Source: CAD feature listing. Evaluate the final solid. Frame: model axes, mm. Face numbers are marked on the shaded views. Coordinates: 2 decimals unless noted, no trailing zeros. Write each loop counter-clockwise with the first axis right and the second up, starting at its lowest first coordinate (ties: lowest second). Pieces come first, ordered by that corner, then holes. Notation, with made-up numbers: (-39.5, -5.75) -> (-30.5, -5.75) arc R16 ccw to (-30.5, 5.25) -> close; hole circle Ø8 at (52.25, 26). An arc over 180 degrees is marked (long way). One line per item, written item: value. Start each with the question number.
1. Section query B-B, the plane z = -12.5. Output: boundary loops of the cut face in (x, y) (3 decimals), and give its area (3 significant figures).
2. Section query A-A, the plane x = 55.4. Output: boundary loops of the cut face in (y, z) (3 decimals), and give its area (3 significant figures).
3. Section query C-C, the plane z = -23. Output: boundary loops of the cut face in (x, y) (3 decimals).
4. Mould query, pull axis Z, two halves, no side actions, for the marked faces 1 and 2. Classes: released by +Z, released by -Z, zero draft, split by the parting line, or undercut.
5. Line query: line 1 (X direction, y = -0.05, z = -74.5); line 2 (X direction, y = -3.5, z = -37); line 3 (Z direction, x = 18, y = -2.5). Output: solid intervals per line, ascending.
6. First-contact query: P1, Ø3.5, axis at x = 30, z = -54.5, coming from the +Y side (3 decimals); P2, Ø10, axis at x = 69, z = -76, coming from the -Y side (3 decimals); P3, Ø3.5, axis at x = 36.9, z = -2.5, coming from the +Y side; P4, Ø2, axis at x = 36.5, z = 3.5, coming from the -Y side (3 decimals). Flat tips, straight axial feed; report the tip coordinate or a pass-through.
from build123d import *

# Parameters (mm, degrees)
SKETCH1_W           = 85.8
SKETCH1_H           = 92.5
SKETCH1_R           = 2.05
BOSS_EXTRUDE1_DEPTH = 3.175
SKETCH2_W           = 85.8
SKETCH2_H           = 92.5
SKETCH2_R           = 1.35
SKETCH2_R_2         = 3.35
BOSS_EXTRUDE2_DEPTH = 1.905
BOSS_EXTRUDE3_START = 1
SKETCH2_3_W         = 85.8
SKETCH2_3_H         = 92.5
SKETCH2_3_R         = 1.35
SKETCH2_3_R_2       = 3.35
BOSS_EXTRUDE3_DEPTH = 1
SKETCH3_W           = 85.8
SKETCH3_H           = 92.5
SKETCH3_W_2         = 75.8
SKETCH3_H_2         = 82.5
BOSS_EXTRUDE4_DEPTH = 4.55
SKETCH4_W           = 14
SKETCH4_H           = 6.75
CUT_EXTRUDE1_DEPTH  = 118.864146478
SKETCH5_W           = 10
SKETCH5_H           = 6
CUT_EXTRUDE2_DEPTH  = 118.864146478
BOSS_EXTRUDE5_DEPTH = 5
FILLET1_R           = 2.5
FILLET2_R           = 2.5
FILLET3_R           = 2.5
FILLET4_R           = 2.5
FILLET5_R           = 2.5


with BuildPart() as part:
    # Sketch1 → Boss-Extrude1 (new body)
    with BuildSketch(Plane(origin=(0, 0, 0), x_dir=(1, 0, 0), z_dir=(0, 1, 0))):
        with Locations((36.9, 40.25)):
            Rectangle(SKETCH1_W, SKETCH1_H)
        with Locations(Location((2.5, 12.5, 0), (0, 0, 270))):
            Circle(SKETCH1_R, mode=Mode.SUBTRACT)
        with Locations(Location((18.4, 2.5, 0), (0, 0, 270))):
            Circle(SKETCH1_R, mode=Mode.SUBTRACT)
        with Locations(Location((36.9, 2.5, 0), (0, 0, 270))):
            Circle(SKETCH1_R, mode=Mode.SUBTRACT)
        with Locations(Location((55.4, 2.5, 0), (0, 0, 270))):
            Circle(SKETCH1_R, mode=Mode.SUBTRACT)
        with Locations(Location((29.3, 55.1, 0), (0, 0, 270))):
            Circle(SKETCH1_R, mode=Mode.SUBTRACT)
        with Locations(Location((70.8, 74.5, 0), (0, 0, 270))):
            Circle(SKETCH1_R, mode=Mode.SUBTRACT)
    extrude(amount=BOSS_EXTRUDE1_DEPTH)

    # Sketch2 → Boss-Extrude2 (add)
    # profile 1 of 2: a face of its own
    with BuildSketch(Plane(origin=(0, 0, 0), x_dir=(1, 0, 0), z_dir=(0, 1, 0))):
        with Locations((36.9, 40.25)):
            Rectangle(SKETCH2_W, SKETCH2_H)
        with Locations(Location((2.5, 12.5, 0), (0, 0, 270))):
            Circle(SKETCH2_R, mode=Mode.SUBTRACT)
        with Locations(Location((18.4, 2.5, 0), (0, 0, 270))):
            Circle(SKETCH2_R, mode=Mode.SUBTRACT)
        with Locations(Location((36.9, 2.5, 0), (0, 0, 270))):
            Circle(SKETCH2_R, mode=Mode.SUBTRACT)
        with Locations(Location((55.4, 2.5, 0), (0, 0, 270))):
            Circle(SKETCH2_R, mode=Mode.SUBTRACT)
        with Locations(Location((70.8, 74.5, 0), (0, 0, 270))):
            Circle(SKETCH2_R, mode=Mode.SUBTRACT)
        with BuildLine():
            Line((65.8, 74.5), (65.8, 81.5))
            Line((65.8, 81.5), (-1, 81.5))
            Line((-1, 81.5), (-1, 17.5))
            Line((-1, 17.5), (2.5, 17.5))
            ThreePointArc((2.5, 17.5), (7.5, 12.5), (2.5, 7.5))
            Line((2.5, 7.5), (-1, 7.5))
            Line((-1, 7.5), (-1, -1))
            Line((-1, -1), (13.4, -1))
            Line((13.4, -1), (13.4, 2.5))
            ThreePointArc((13.4, 2.5), (18.4, 7.5), (23.4, 2.5))
            Line((23.4, 2.5), (23.4, -1))
            Line((23.4, -1), (31.9, -1))
            Line((31.9, -1), (31.9, 2.5))
            ThreePointArc((31.9, 2.5), (36.9, 7.5), (41.9, 2.5))
            Line((41.9, 2.5), (41.9, -1))
            Line((41.9, -1), (50.4, -1))
            Line((50.4, -1), (50.4, 2.5))
            ThreePointArc((50.4, 2.5), (55.4, 7.5), (60.4, 2.5))
            Line((60.4, 2.5), (60.4, -1))
            Line((60.4, -1), (74.8, -1))
            Line((74.8, -1), (74.8, 69.5))
            Line((74.8, 69.5), (70.8, 69.5))
            ThreePointArc((70.8, 69.5), (67.264466094, 70.964466094), (65.8, 74.5))
        make_face(mode=Mode.SUBTRACT)
    # profile 2 of 2: a face of its own
    with BuildSketch(Plane(origin=(0, 0, 0), x_dir=(1, 0, 0), z_dir=(0, 1, 0))):
        with Locations(Location((29.3, 55.1, 0), (0, 0, 270))):
            Circle(SKETCH2_R_2)
        with Locations(Location((29.3, 55.1, 0), (0, 0, 270))):
            Circle(SKETCH2_R, mode=Mode.SUBTRACT)
    extrude(amount=-BOSS_EXTRUDE2_DEPTH)

    # Sketch2_3 → Boss-Extrude3 (add)
    # profile 1 of 2: a face of its own
    with BuildSketch(Plane(origin=(0, 0, 0), x_dir=(1, 0, 0), z_dir=(0, 1, 0)).offset(BOSS_EXTRUDE3_START)):
        with Locations((36.9, 40.25)):
            Rectangle(SKETCH2_3_W, SKETCH2_3_H)
        with Locations(Location((2.5, 12.5, 0), (0, 0, 270))):
            Circle(SKETCH2_3_R, mode=Mode.SUBTRACT)
        with Locations(Location((18.4, 2.5, 0), (0, 0, 270))):
            Circle(SKETCH2_3_R, mode=Mode.SUBTRACT)
        with Locations(Location((36.9, 2.5, 0), (0, 0, 270))):
            Circle(SKETCH2_3_R, mode=Mode.SUBTRACT)
        with Locations(Location((55.4, 2.5, 0), (0, 0, 270))):
            Circle(SKETCH2_3_R, mode=Mode.SUBTRACT)
        with Locations(Location((70.8, 74.5, 0), (0, 0, 270))):
            Circle(SKETCH2_3_R, mode=Mode.SUBTRACT)
        with BuildLine():
            Line((65.8, 74.5), (65.8, 81.5))
            Line((65.8, 81.5), (-1, 81.5))
            Line((-1, 81.5), (-1, 17.5))
            Line((-1, 17.5), (2.5, 17.5))
            ThreePointArc((2.5, 17.5), (7.5, 12.5), (2.5, 7.5))
            Line((2.5, 7.5), (-1, 7.5))
            Line((-1, 7.5), (-1, -1))
            Line((-1, -1), (13.4, -1))
            Line((13.4, -1), (13.4, 2.5))
            ThreePointArc((13.4, 2.5), (18.4, 7.5), (23.4, 2.5))
            Line((23.4, 2.5), (23.4, -1))
            Line((23.4, -1), (31.9, -1))
            Line((31.9, -1), (31.9, 2.5))
            ThreePointArc((31.9, 2.5), (36.9, 7.5), (41.9, 2.5))
            Line((41.9, 2.5), (41.9, -1))
            Line((41.9, -1), (50.4, -1))
            Line((50.4, -1), (50.4, 2.5))
            ThreePointArc((50.4, 2.5), (55.4, 7.5), (60.4, 2.5))
            Line((60.4, 2.5), (60.4, -1))
            Line((60.4, -1), (74.8, -1))
            Line((74.8, -1), (74.8, 69.5))
            Line((74.8, 69.5), (70.8, 69.5))
            ThreePointArc((70.8, 69.5), (67.264466094, 70.964466094), (65.8, 74.5))
        make_face(mode=Mode.SUBTRACT)
    # profile 2 of 2: a face of its own
    with BuildSketch(Plane(origin=(0, 0, 0), x_dir=(1, 0, 0), z_dir=(0, 1, 0)).offset(BOSS_EXTRUDE3_START)):
        with Locations(Location((29.3, 55.1, 0), (0, 0, 270))):
            Circle(SKETCH2_3_R_2)
        with Locations(Location((29.3, 55.1, 0), (0, 0, 270))):
            Circle(SKETCH2_3_R, mode=Mode.SUBTRACT)
    extrude(amount=-BOSS_EXTRUDE3_DEPTH)

    # Sketch3 → Boss-Extrude4 (add)
    with BuildSketch(Plane(origin=(0, -1.905, 0), x_dir=(-1, 0, 0), z_dir=(0, -1, 0))):
        with Locations((-36.9, 40.25)):
            Rectangle(SKETCH3_W, SKETCH3_H)
        with Locations((-36.9, 40.25)):
            Rectangle(SKETCH3_W_2, SKETCH3_H_2, mode=Mode.SUBTRACT)
    extrude(amount=BOSS_EXTRUDE4_DEPTH)

    # Sketch4 → Cut-Extrude1 (cut, through all)
    with BuildSketch(Plane.XY):
        with Locations((9.15, -6.47)):
            Rectangle(SKETCH4_W, SKETCH4_H)
        with Locations((27.65, -6.47)):
            Rectangle(SKETCH4_W, SKETCH4_H)
        with Locations((46.15, -6.47)):
            Rectangle(SKETCH4_W, SKETCH4_H)
        with Locations((64.65, -6.47)):
            Rectangle(SKETCH4_W, SKETCH4_H)
    extrude(amount=CUT_EXTRUDE1_DEPTH, mode=Mode.SUBTRACT)

    # Sketch5 → Cut-Extrude2 (cut, through all)
    with BuildSketch(Plane.XY):
        with Locations((58, -7.455)):
            Rectangle(SKETCH5_W, SKETCH5_H)
    extrude(amount=-CUT_EXTRUDE2_DEPTH, mode=Mode.SUBTRACT)

    # Sketch6 → Boss-Extrude5 (add)
    with BuildSketch(Plane.ZY.offset(6)):
        with BuildLine():
            Line((-59.6, 0), (-59.6, -8.95))
            Line((-59.6, -8.95), (-59.131128874, -8.95))
            ThreePointArc((-59.131128874, -8.95), (-55.1, -6.45), (-51.068871126, -8.95))
            Line((-51.068871126, -8.95), (-50.6, -8.95))
            Line((-50.6, -8.95), (-50.6, 0))
            Line((-50.6, 0), (-59.6, 0))
        make_face()
    extrude(amount=-BOSS_EXTRUDE5_DEPTH)

    # Fillet1
    fillet1_edges = [part.edges().sort_by_distance(p)[0] for p in [
        (79.8, -1.64, 6),
    ]]
    fillet(fillet1_edges, radius=FILLET1_R)

    # Fillet2
    fillet2_edges = [part.edges().sort_by_distance(p)[0] for p in [
        (79.8, -1.64, -86.5),
    ]]
    fillet(fillet2_edges, radius=FILLET2_R)

    # Fillet3
    fillet3_edges = [part.edges().sort_by_distance(p)[0] for p in [
        (-6, -1.64, -86.5),
    ]]
    fillet(fillet3_edges, radius=FILLET3_R)

    # Fillet4
    fillet4_edges = [part.edges().sort_by_distance(p)[0] for p in [
        (-6, -1.64, 6),
    ]]
    fillet(fillet4_edges, radius=FILLET4_R)

    # Fillet5
    fillet5_edges = [part.edges().sort_by_distance(p)[0] for p in [
        (79.8, 3.175, -40.25),
        (79.067766953, 3.175, 5.267766953),
        (36.9, 3.175, -86.5),
        (79.067766953, 3.175, -85.767766953),
        (-6, 3.175, -40.25),
        (-5.267766953, 3.175, -85.767766953),
        (36.9, 3.175, 6),
        (-5.267766953, 3.175, 5.267766953),
    ]]
    fillet(fillet5_edges, radius=FILLET5_R)


solid = part.part
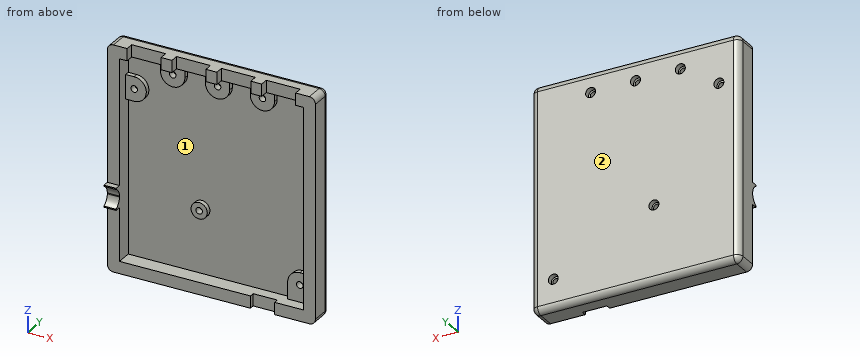
Computed values:
1. outline: (-6, -6.455) -> (-1, -6.455) -> (-1, -1.905) -> (1.15, -1.905) -> (1.15, 1) -> (0.45, 1) -> (0.45, 3.175) -> (-3.5, 3.175) arc R2.5 ccw to (-6, 0.675) -> close; (3.85, -1.905) -> (7.5, -1.905) -> (7.5, 0) -> (74.8, 0) -> (74.8, -6.455) -> (79.8, -6.455) -> (79.8, 0.675) arc R2.5 ccw to (77.3, 3.175) -> (4.55, 3.175) -> (4.55, 1) -> (3.85, 1) -> close
1. area: 334 mm²
2. outline: (-6.455, 1) -> (-1.905, 1) -> (-1.905, -1.15) -> (1, -1.15) -> (1, -0.45) -> (3.175, -0.45) -> (3.175, 3.5) arc R2.5 ccw to (0.675, 6) -> (-6.455, 6) -> close; (-4.455, -86.5) -> (0.675, -86.5) arc R2.5 ccw to (3.175, -84) -> (3.175, -4.55) -> (1, -4.55) -> (1, -3.85) -> (-1.905, -3.85) -> (-1.905, -7.5) -> (0, -7.5) -> (0, -81.5) -> (-4.455, -81.5) -> close
2. area: 345 mm²
3. outline: (-6, -6.455) -> (-1, -6.455) -> (-1, 0) -> (74.8, 0) -> (74.8, -6.455) -> (79.8, -6.455) -> (79.8, 0.675) arc R2.5 ccw to (77.3, 3.175) -> (-3.5, 3.175) arc R2.5 ccw to (-6, 0.675) -> close
4. face 1: undercut
4. face 2: zero draft
5. line 1: x = -6 to -1, 65.8 to 69.45, 72.15 to 79.8
5. line 2: x = -6 to -1, 74.8 to 79.8
5. line 3: z = -86.5 to -81.5, 1 to 6
6. P1: stops at y = 3.175
6. P2: stops at y = -1.905
6. P3: stops at y = 1
6. P4: stops at y = -6.455
